```python
from build123d import *

# Parameters (mm, degrees)
F_3_8_NPT_TAPPED_HOLE1_AT_2_COUNT = 2
F_3_8_NPT_TAPPED_HOLE1_AT_2_PITCH = 76.2


with BuildPart() as part:
    # Sketch1 → Revolve1 (revolve)
    with BuildSketch(Plane.XY):
        Polygon((0, 0), (-76.2, 0), (-76.2, -38.1), (-60.96, -38.1), (-60.96, -32.258), (-55.7149, -32.258), (-51.6509, -32.258), (-32.163982831, -32.258), (-30.364664072, -32.258), (-28.575, -32.258), (-28.575, -27.178), (-28.0924, -27.178), (-24.0284, -27.178), (-22.225, -27.178), (0, -15.85722), align=None)
    revolve(axis=Axis((0, 0, 0), (0, -1, 0)))

    # Sketch3 → 1/2 NPT Tapped Hole1 (revolve, cut)
    with BuildSketch(Plane(origin=(0, 0, 0), x_dir=(0, 0, 1), z_dir=(1, 0, 0))):
        Polygon((0, 0), (0, 38.1), (8.9281, 38.1), (8.9281, 13.462), (10.261665792, 13.462), (10.6647361, 0), align=None)
    revolve(axis=Axis((0, 6.35, 0), (0, -1, 0)), mode=Mode.SUBTRACT)

    # Sketch5 → 3/8 NPT Tapped Hole1 (revolve, cut)
    with BuildSketch(Plane(origin=(-38.1, 0, 0), x_dir=(0, 0, 1), z_dir=(1, 0, 0))):
        Polygon((0, 0), (0, 38.1), (7.1374, 38.1), (7.1374, 10.414), (8.263205494, 10.414), (8.5750146, 0), align=None)
    f_3_8_npt_tapped_hole1 = revolve(axis=Axis((-38.1, 6.35, 0), (0, -1, 0)), mode=Mode.SUBTRACT)

    # 3/8 NPT Tapped Hole1 at 2: 3/8 NPT Tapped Hole1 ×2
    with Locations(*[(i * F_3_8_NPT_TAPPED_HOLE1_AT_2_PITCH, 0, 0) for i in range(1, F_3_8_NPT_TAPPED_HOLE1_AT_2_COUNT)]):
        add(f_3_8_npt_tapped_hole1, mode=Mode.SUBTRACT)


solid = part.part
```
For this review, take the finished solid that the model builds, in its own axes (mm). A direction names the side the tool comes from. Round coordinates to 2 decimals unless told otherwise and drop trailing zeros. Write each loop counter-clockwise with the first axis right and the second up, starting at its lowest first coordinate (ties: lowest second). Pieces come first, ordered by that corner, then holes. Notation, with made-up numbers: (-37.75, -20.5) -> (-0.75, -20.5) arc R10 ccw to (-0.75, -14.5) -> close; hole circle Ø6 at (14, 21). An arc over 180 degrees is marked (long way). One line per question, with ' | ' between items. Start each with the question number.
(1) Add section A-A, the plane x = -38.1. Write out the cut boundary in (y, z).
(2) Add section B-B, the plane z = 0. Give the number of separate pieces and of enclosed holes in the cut face, plus the area to 3 significant figures.
(3) Mouldability with a two-part tool opening along Z and no side actions: class faces 1 (the face through (34, -38.1, -51)), 2 (the face through (60.47, -19.317, 46.367)), 3 (the face through (6.368, -6.637, -8.305)), 4 (the face through (45.068, -21.183, -1.547)) as released by +Z, released by -Z, zero draft, split by the parting line, or undercut.
(4) Insertion check: P1, Ø6, axis at y = -26, z = -51.5, coming from the +X side; P2, Ø8, axis at y = -10, z = -45, coming from the -X side; P3, Ø14.5, axis at x = 0, z = 0, coming from the -Y side; P4, Ø18.5, axis at x = -38.1, z = 0, coming from the -Y side. Each pin has a flat end and moves straight along its axis. Give the tip position at first contact, or say it passes through.
(5) For line 1 along X through (y, z) = (-29, 0) (3 decimals); line 2 along Z through (x, y) = (0, -30.1) (3 decimals); line 3 along X through (y, z) = (-27, 0), list the stretches that pass through material, from the lowest coordinate up. Write a range as from..to.
(6) Tool access review of faces 5 (the face through (41, -10.414, 7)), 6 (the face through (-31.132, -21.183, -1.547)), 7 (the face through (-15, -27.178, 17)): name each direction out of +Z, -Z, +X, -X, +Y, -Y from which nothing blocks a thin tool from reaching the whole face with its end or side.
(7) Add section D-D, the plane z = 54. Write out the cut boundary in (x, y).
(8) Add section C-C, the plane y = -16. Write out the cut boundary in (x, z).
Answer list:
1) outline: (-38.1, -65.99) -> (0, -65.99) -> (0, -8.58) -> (-10.41, -8.26) -> (-10.41, -7.14) -> (-32.26, -7.14) -> (-32.26, -47.59) -> (-38.1, -47.59) -> close; (-38.1, 47.59) -> (-32.26, 47.59) -> (-32.26, 7.14) -> (-10.41, 7.14) -> (-10.41, 8.26) -> (0, 8.58) -> (0, 65.99) -> (-38.1, 65.99) -> close
2) separate pieces: 4 | enclosed holes: 0 | area: 3,210 mm²
3) face 1: zero draft | face 2: split by the parting line | face 3: undercut | face 4: undercut
4) P1: x = 58.77 | P2: x = -64.23 | P3: through | P4: y = -32.26
5) line 1: -76.2..-45.237, -30.963..-28.575, 28.575..30.963, 45.237..76.2 | line 2: -76.2..-28.575, 28.575..76.2 | line 3: -76.2..-45.24, -30.96..-21.88, 21.88..30.96, 45.24..76.2
6) face 5: +Y | face 6: +Y, -Y | face 7: -Y
7) outline: (-53.76, -38.1) -> (-28.29, -38.1) -> (-28.29, -32.26) -> (28.29, -32.26) -> (28.29, -38.1) -> (53.76, -38.1) -> (53.76, 0) -> (-53.76, 0) -> close
8) outline: circle Ø152.4 at (0, 0); hole circle Ø14.27 at (-38.1, 0); hole circle Ø17.86 at (0, 0); hole circle Ø14.27 at (38.1, 0)
